Autodesk Inventor part; units mm, degrees
ref_plane "YZ Plane" through (0, 0, 0) normal (1, 0, 0) x (0, 1, 0)
ref_plane "XZ Plane" through (0, 0, 0) normal (0, 1, 0) x (-1, 0, 0)
ref_plane "XY Plane" through (0, 0, 0) normal (0, 0, 1) x (1, 0, 0)
sketch "Sketch1" plane through (0, 0, 0) normal (0, 0, 1) x (1, 0, 0)
  circle A0 centre (0, 0) radius 15.025
  dimension "d0" = 30.05
extrude "Extrusion1" add sketch "Sketch1" along normal blind 7.1
sketch "Sketch2" plane through (0, 0, 7.1) normal (0, 0, 1) x (1, 0, 0)
  circle A0 centre (0, 0) radius 16
  dimension "d3" = 32
extrude "Extrusion2" add sketch "Sketch2" along normal blind 1
sketch "Sketch3" plane through (0, 0, 8.1) normal (0, 0, 1) x (1, 0, 0)
  circle A0 centre (0, 0) radius 20
  dimension "d6" = 40
extrude "Extrusion3" add sketch "Sketch3" along normal blind 4
sketch "Sketch4" plane through (0, 0, 0) normal (0, 0, -1) x (-1, 0, 0)
  circle A0 centre (0, 0) radius 16
  line L0 (6, 25.2369) -> (-6, 25.2369)
  line L1 (-6, 25.2369) -> (-6, -24.7248)
  line L2 (-6, -24.7248) -> (6, -24.7248)
  line L3 (6, -24.7248) -> (6, 25.2369)
  point P0 (6, -14.8324)
  point P1 (6, 14.8324)
  point P2 (-6, 14.8324)
  point P3 (-6, -14.8324)
  dimension "d9" = 6
  dimension "d10" = 6
extrude "Extrusion4" cut sketch "Sketch4" against normal through all contours L3 A0 L1
chamfer "Chamfer1" distance 7 angle 45 2 edges at (-6, 0, 0) (6, 0, 0)
chamfer "Chamfer3" distance 1 angle 45 2 edges at (-20, 0, 8.1) (-20, 0, 12.1)
sketch "Sketch6" plane through (0, 0, 12.1) normal (0, 0, 1) x (1, 0, 0)
  circle A0 centre (-12.5, -5) radius 1.55
  arc A1 (-13, 7.5333) -> (-13, -7.5333) centre (0, 0) ccw
  line L0 (-13, -7.5333) -> (-13, 7.5333)
  line L1 (0, 0) -> (0, -4.0369)
  line L2 (0, 0) -> (-1.7679, 0)
  circle A2 centre (12.5, -5) radius 1.55
  circle A3 centre (-12.5, 5) radius 1.55
  circle A4 centre (12.5, 5) radius 1.55
  dimension "d22" = 5
  dimension "d23" = 12.5
  dimension "d24" = 3.1
extrude "Extrusion5" cut sketch "Sketch6" against normal through all contours A0 L0 | L0 A0 | A3 L0 | L0 A3 | A2 | A4
sketch "Sketch7" plane through (0, 0, 12.1) normal (0, 0, 1) x (1, 0, 0)
  circle A0 centre (-12.5, -5) radius 1.55
  circle A1 centre (-12.5, 5) radius 1.55
  circle A2 centre (12.5, 5) radius 1.55
  circle A3 centre (12.5, -5) radius 1.55
  circle A4 centre (-12.5, -5) radius 3
  circle A5 centre (-12.5, 5) radius 3
  circle A6 centre (12.5, 5) radius 3
  circle A7 centre (12.5, -5) radius 3
  point P0 (0, 0)
  dimension "d27" = 6
  dimension "d28" = 6
  dimension "d29" = 6
  dimension "d30" = 6
extrude "Extrusion6" cut sketch "Sketch7" against normal blind 2
chamfer "Chamfer4" distance 1.4 angle 45 4 edges at (-14.05, -5, 10.1) (-14.05, 5, 10.1) (10.95, 5, 10.1) (10.95, -5, 10.1)
chamfer "Chamfer5" distance 0.2 angle 45 4 edges at (-15.5, -5, 12.1) (-15.5, 5, 12.1) (9.5, -5, 12.1) (9.5, 5, 12.1)
chamfer "Chamfer8" distance 3.6 angle 45 2 edges at (-6, 0, 7) (6, 0, 7)
equation "\"d28\" = d27"
equation "\"d29\" = d27"
equation "\"d30\" = d27"
properties part number "arm_head"
Geometry check sheet. Reference: the model listing, model coordinates, mm. A direction names the side the tool comes from. Coordinates: 2 decimals unless noted, no trailing zeros. Order: outer loops, then holes, each group sorted by start corner. A loop starts at its lowest first (then second) coordinate and runs counter-clockwise, first axis right, second up. Notation, with made-up numbers: (35.25, -9.5) - (70.25, -9.5) arc R32 cw to (70.25, 18.5) - close; hole circle Ø3 at (-1, 2). An arc over 180 degrees is marked (long way). Answer in a Markdown table with one row per item. Add a question column.
1. Access from +Z, -Z, +X, -X, +Y, -Y to the whole of each face (thin tool, end or side, straight path). Record for faces 1 (the face through (-14.9, 3.2, 11)), 2 (the face through (7.255, 0.208, 7.57)), 3 (the face through (6, 0, 11)), 4 (the face through (15.2, 0.1, 7.1)).
2. Section check A-A (y = 0). Enter the section's corners in (x, z) (3 decimals).
3. Section check B-B (x = 0). Enter the section's corners in (y, z), plus the area to 3 significant figures.
4. Material ranges on L1, parallel to Y at x = 11, z = 10.5; L2, parallel to X at y = -5, z = 7.25; L3, parallel to Y at x = 12.5, z = 11.1, recorded low to high. Write a range as [from, to].
5. Section check D-D (x = 12.5). Give the number of separate pieces and of enclosed holes in the cut face, plus the area to 3 significant figures.
6. Section check C-C (z = 6.25). Enter the section's corners in (x, y) (3 decimals), plus the area to 3 significant figures.
7. Gauge pin test, flat ends, axial feed: pin 1 Ø3 at (x, z) = (10.5, 6.5) entering from +Y; pin 2 Ø5 at (x, y) = (-12.5, 5) entering from +Z; pin 3 Ø0.8 at (y, z) = (-5.5, 11.5) entering from +X; pin 4 Ø1.9 at (x, y) = (12.5, -5) entering from -Z. Record the tip position at first contact, or that the pin passes through.
Data:
| question | item | result |
|---|---|---|
| 1 | face 1 | +Z |
| 1 | face 2 | -Z |
| 1 | face 3 | +Z, -Z |
| 1 | face 4 | -Z, +X |
| 2 | outline | (-20, 9.1) - (-19, 8.1) - (-16, 8.1) - (-16, 7.1) - (-15.025, 7.1) - (-15.025, 0) - (-13, 0) - (-8.546, 4.454) - (-6, 10.6) - (-6, 12.1) - (-19, 12.1) - (-20, 11.1) - close; (6, 10.6) - (8.546, 4.454) - (13, 0) - (15.025, 0) - (15.025, 7.1) - (16, 7.1) - (16, 8.1) - (19, 8.1) - (20, 9.1) - (20, 11.1) - (19, 12.1) - (6, 12.1) - close |
| 3 | outline | (-20, 9.1) - (-19, 8.1) - (-16, 8.1) - (-16, 12.1) - (-19, 12.1) - (-20, 11.1) - close; (16, 8.1) - (19, 8.1) - (20, 9.1) - (20, 11.1) - (19, 12.1) - (16, 12.1) - close |
| 3 | area | 30.0 mm² |
| 4 | L1 | y = [-16.7, -7.6], [-2.4, 2.4], [7.6, 16.7] |
| 4 | L2 | x = [-15.2, -14.05], [-10.95, -7.39], [7.39, 10.95], [14.05, 15.2] |
| 4 | L3 | y = [-15.61, -8], [-2, 2], [8, 15.61] |
| 5 | separate pieces | 3 |
| 5 | enclosed holes | 0 |
| 5 | area | 165 mm² |
| 6 | outline | (-7.802, -12.841) - (-7.802, 12.841) arc R15.025 ccw to start; (7.802, -12.841) arc R15.025 ccw to (7.802, 12.841) - close; hole circle Ø3.1 at (-12.5, -5); hole circle Ø3.1 at (-12.5, 5); hole circle Ø3.1 at (12.5, -5); hole circle Ø3.1 at (12.5, 5) |
| 6 | area | 232 mm² |
| 7 | pin 1 | stops at y = 13.14 |
| 7 | pin 2 | stops at z = 9.65 |
| 7 | pin 3 | stops at x = 19.24 |
| 7 | pin 4 | passes through |
